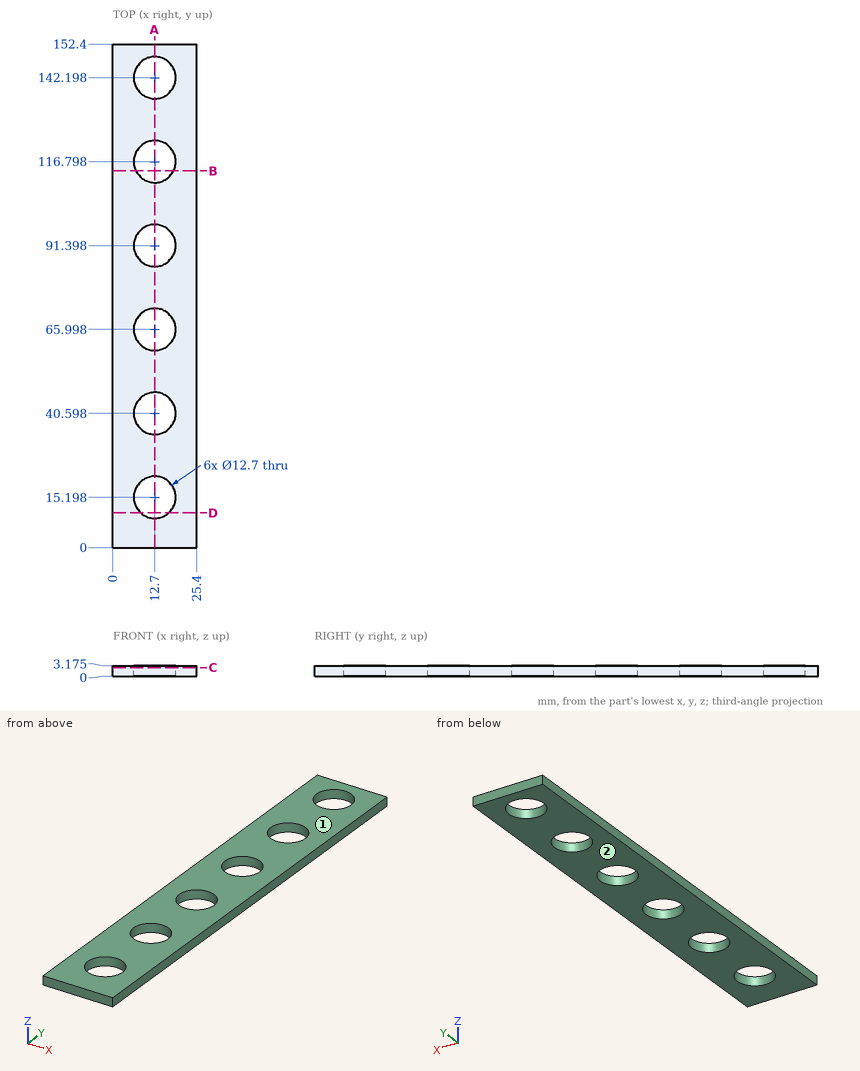
Geometry check sheet. Reference: drawing and pictorial views, mm from the part's lowest x, y, z. Coordinates: 2 decimals unless noted, no trailing zeros. Order: outer loops, then holes, each group sorted by start corner. A loop starts at its lowest first (then second) coordinate and runs counter-clockwise, first axis right, second up. Notation, with made-up numbers: (78.25, 4.25) -> (106.25, 4.25) arc R10 ccw to (106.25, 21.25) -> close; hole circle Ø5 at (89.25, -14). An arc over 180 degrees is marked (long way). Put each result on its own line as item: value. Start each with the question number.
1) Cross-section at D-D (y = 10.5). Enter the section's corners in (x, z) (1 decimal), plus the area to 3 significant figures.
2) Material ranges on L1, parallel to X at y = 46, z = 0.65; L2, parallel to X at y = 86.5, z = 0.9, recorded low to high.
3) Release check for a two-part mould opening along Z. For the marked faces 1 and 2 record: pulls with the +Z half, pulls with the -Z half, needs draft (parallel to the pull), parting line crosses it, or undercut.
4) Cross-section at C-C (z = 2.55). Enter the section's corners in (x, y).
5) Cross-section at B-B (y = 114). Enter the section's corners in (x, z) (1 decimal).
6) Cross-section at A-A (x = 12.7). Enter the section's corners in (y, z) (1 decimal), plus the area to 3 significant figures.
7) Go/stop test with a flat-tipped pin: pin 1 (10 mm diameter, centred on x = 12.7, y = 40.6, fed in from +Z). Record where the tip stops, or that it passes through.
Geometry check:
1. outline: (0, 0) -> (8.4, 0) -> (8.4, 3.2) -> (0, 3.2) -> close; (17, 0) -> (25.4, 0) -> (25.4, 3.2) -> (17, 3.2) -> close
1. area: 53.5 mm^2
2. L1: x = 0 to 9.36, 16.04 to 25.4
2. L2: x = 0 to 8.66, 16.74 to 25.4
3. face 1: pulls with the +Z half
3. face 2: pulls with the -Z half
4. outline: (0, 0) -> (25.4, 0) -> (25.4, 152.4) -> (0, 152.4) -> close; hole circle Ø12.7 at (12.7, 15.2); hole circle Ø12.7 at (12.7, 40.6); hole circle Ø12.7 at (12.7, 66); hole circle Ø12.7 at (12.7, 91.4); hole circle Ø12.7 at (12.7, 116.8); hole circle Ø12.7 at (12.7, 142.2)
5. outline: (0, 0) -> (7, 0) -> (7, 3.2) -> (0, 3.2) -> close; (18.4, 0) -> (25.4, 0) -> (25.4, 3.2) -> (18.4, 3.2) -> close
6. outline: (0, 0) -> (8.8, 0) -> (8.8, 3.2) -> (0, 3.2) -> close; (21.5, 0) -> (34.2, 0) -> (34.2, 3.2) -> (21.5, 3.2) -> close; (46.9, 0) -> (59.6, 0) -> (59.6, 3.2) -> (46.9, 3.2) -> close; (72.3, 0) -> (85, 0) -> (85, 3.2) -> (72.3, 3.2) -> close; (97.7, 0) -> (110.4, 0) -> (110.4, 3.2) -> (97.7, 3.2) -> close; (123.1, 0) -> (135.8, 0) -> (135.8, 3.2) -> (123.1, 3.2) -> close; (148.5, 0) -> (152.4, 0) -> (152.4, 3.2) -> (148.5, 3.2) -> close
6. area: 242 mm^2
7. pin 1: passes through
